Work out the finished part from the listing and answer in its coordinate system (mm). Face numbers are marked on the shaded views. Coordinates: 2 decimals unless noted, no trailing zeros. Order: outer loops, then holes, each group sorted by start corner. A loop starts at its lowest first (then second) coordinate and runs counter-clockwise, first axis right, second up. Notation, with made-up numbers: (71.25, -39.5) - (114.25, -39.5) arc R31 ccw to (114.25, -10.5) - close; hole circle Ø1 at (3.5, 16). An arc over 180 degrees is marked (long way). Answer as a JSON object with one key per item and string values. Group by question number.
1) Find the intervals of material crossed by line 1 along Y through (x, z) = (94.15, 13.65); line 2 along X through (y, z) = (-47, 10.75); line 3 along Y through (x, z) = (-94.15, 6.5), in increasing order.
2) Each of these flat-tipped pins is pushed along its axis until it touches: P1, Ø2, axis at x = -94.5, y = 53, coming from the +Z side; P2, Ø12, axis at x = 78, y = -17.5, coming from the -Z side; P3, Ø6.5, axis at x = 94.15, y = -54, coming from the -Z side. Where does it stop, or does it pass through?
3) Section C-C (z = 8) is taken. Count the separate pieces of the cut face and the enclosed holes in it, plus the area to 3 significant figures.
4) Section B-B (y = -26) is taken. Give the vertices of the cut face in (x, z).
5) Section A-A (x = 37) is taken. Give the vertices of the cut face in (y, z), plus the area to 3 significant figures.
6) The mould has two halves that part along X. Classify the marked faces 1 and 2: released by +X, released by -X, zero draft, split by the parting line, or undercut.
from build123d import *

# Parameters (mm, degrees)
SKETCH1_R           = 2
BOSS_EXTRUDE1_DEPTH = 15.2
SKETCH2_R           = 3.75
CUT_EXTRUDE1_DEPTH  = 2.9
FILLET1_R           = 1
CUT_EXTRUDE2_DEPTH  = 11.2
BOSS_EXTRUDE2_DEPTH = 1
CUT_EXTRUDE3_DEPTH  = 2.5
CUT_EXTRUDE4_DEPTH  = 11.2


with BuildPart() as part:
    # Sketch1 → Boss-Extrude1 (new body)
    with BuildSketch(Plane.XY):
        with BuildLine():
            Line((-95, -60), (95, -60))
            ThreePointArc((95, -60), (98.535533906, -58.535533906), (100, -55))
            Line((100, -55), (100, 55))
            ThreePointArc((100, 55), (98.535533906, 58.535533906), (95, 60))
            Line((95, 60), (-95, 60))
            ThreePointArc((-95, 60), (-98.535533906, 58.535533906), (-100, 55))
            Line((-100, 55), (-100, -55))
            ThreePointArc((-100, -55), (-98.535533906, -58.535533906), (-95, -60))
        make_face()
        with Locations((94.15, -54)):
            Circle(SKETCH1_R, mode=Mode.SUBTRACT)
        with Locations((94.15, 54)):
            Circle(SKETCH1_R, mode=Mode.SUBTRACT)
        with Locations((-94.15, 54)):
            Circle(SKETCH1_R, mode=Mode.SUBTRACT)
        with Locations((-94.15, -54)):
            Circle(SKETCH1_R, mode=Mode.SUBTRACT)
    extrude(amount=BOSS_EXTRUDE1_DEPTH)

    # Sketch2 → Cut-Extrude1 (cut)
    with BuildSketch(Plane.XY.offset(15.2)):
        with Locations((-94.15, 54)):
            Circle(SKETCH2_R)
        with Locations((94.15, 54)):
            Circle(SKETCH2_R)
        with Locations((94.15, -54)):
            Circle(SKETCH2_R)
        with Locations((-94.15, -54)):
            Circle(SKETCH2_R)
    extrude(amount=-CUT_EXTRUDE1_DEPTH, mode=Mode.SUBTRACT)

    # Fillet1
    fillet1_edges = [part.edges().sort_by_distance(p)[0] for p in [
        (98.535533906, -58.535533906, 15.2),
        (100, 0, 15.2),
        (98.535533906, 58.535533906, 15.2),
        (0, 60, 15.2),
        (-98.535533906, 58.535533906, 15.2),
        (-100, 0, 15.2),
        (-98.535533906, -58.535533906, 15.2),
        (0, -60, 15.2),
    ]]
    fillet(fillet1_edges, radius=FILLET1_R)

    # Sketch3 → Cut-Extrude2 (cut)
    with BuildSketch(Plane(origin=(0, 0, 0), x_dir=(-1, 0, 0), z_dir=(0, 0, -1))):
        with BuildLine():
            Line((86.35, -52.7), (86.35, -42.7))
            ThreePointArc((86.35, -42.7), (87.960912703, -38.810912703), (91.85, -37.2))
            Line((91.85, -37.2), (92.7, -37.2))
            ThreePointArc((92.7, -37.2), (94.467766953, -36.467766953), (95.2, -34.7))
            Line((95.2, -34.7), (95.2, 34.7))
            ThreePointArc((95.2, 34.7), (94.467766953, 36.467766953), (92.7, 37.2))
            Line((92.7, 37.2), (91.85, 37.2))
            ThreePointArc((91.85, 37.2), (87.960912703, 38.810912703), (86.35, 42.7))
            Line((86.35, 42.7), (86.35, 52.7))
            ThreePointArc((86.35, 52.7), (85.617766953, 54.467766953), (83.85, 55.2))
            Line((83.85, 55.2), (-83.85, 55.2))
            ThreePointArc((-83.85, 55.2), (-85.617766953, 54.467766953), (-86.35, 52.7))
            Line((-86.35, 52.7), (-86.35, 42.7))
            ThreePointArc((-86.35, 42.7), (-87.960912703, 38.810912703), (-91.85, 37.2))
            Line((-91.85, 37.2), (-92.7, 37.2))
            ThreePointArc((-92.7, 37.2), (-94.467766953, 36.467766953), (-95.2, 34.7))
            Line((-95.2, 34.7), (-95.2, -34.7))
            ThreePointArc((-95.2, -34.7), (-94.467766953, -36.467766953), (-92.7, -37.2))
            Line((-92.7, -37.2), (-91.85, -37.2))
            ThreePointArc((-91.85, -37.2), (-87.960912703, -38.810912703), (-86.35, -42.7))
            Line((-86.35, -42.7), (-86.35, -52.7))
            ThreePointArc((-86.35, -52.7), (-85.617766953, -54.467766953), (-83.85, -55.2))
            Line((-83.85, -55.2), (83.85, -55.2))
            ThreePointArc((83.85, -55.2), (85.617766953, -54.467766953), (86.35, -52.7))
        make_face()
    extrude(amount=-CUT_EXTRUDE2_DEPTH, mode=Mode.SUBTRACT)

    # Sketch4 → Boss-Extrude2 (add)
    with BuildSketch(Plane(origin=(0, 0, 0), x_dir=(-1, 0, 0), z_dir=(0, 0, -1))):
        with BuildLine():
            Line((-83.85, -56.2), (83.85, -56.2))
            ThreePointArc((83.85, -56.2), (86.324873734, -55.174873734), (87.35, -52.7))
            Line((87.35, -52.7), (87.35, -42.7))
            ThreePointArc((87.35, -42.7), (88.668019485, -39.518019485), (91.85, -38.2))
            Line((91.85, -38.2), (92.7, -38.2))
            ThreePointArc((92.7, -38.2), (95.174873734, -37.174873734), (96.2, -34.7))
            Line((96.2, -34.7), (96.2, 34.7))
            ThreePointArc((96.2, 34.7), (95.174873734, 37.174873734), (92.7, 38.2))
            Line((92.7, 38.2), (91.85, 38.2))
            ThreePointArc((91.85, 38.2), (88.668019485, 39.518019485), (87.35, 42.7))
            Line((87.35, 42.7), (87.35, 52.7))
            ThreePointArc((87.35, 52.7), (86.324873734, 55.174873734), (83.85, 56.2))
            Line((83.85, 56.2), (-83.85, 56.2))
            ThreePointArc((-83.85, 56.2), (-86.324873734, 55.174873734), (-87.35, 52.7))
            Line((-87.35, 52.7), (-87.35, 42.7))
            ThreePointArc((-87.35, 42.7), (-88.668019485, 39.518019485), (-91.85, 38.2))
            Line((-91.85, 38.2), (-92.7, 38.2))
            ThreePointArc((-92.7, 38.2), (-95.174873734, 37.174873734), (-96.2, 34.7))
            Line((-96.2, 34.7), (-96.2, -34.7))
            ThreePointArc((-96.2, -34.7), (-95.174873734, -37.174873734), (-92.7, -38.2))
            Line((-92.7, -38.2), (-91.85, -38.2))
            ThreePointArc((-91.85, -38.2), (-88.668019485, -39.518019485), (-87.35, -42.7))
            Line((-87.35, -42.7), (-87.35, -52.7))
            ThreePointArc((-87.35, -52.7), (-86.324873734, -55.174873734), (-83.85, -56.2))
        make_face()
        with BuildLine():
            Line((86.35, -52.7), (86.35, -42.7))
            ThreePointArc((86.35, -42.7), (87.960912703, -38.810912703), (91.85, -37.2))
            Line((91.85, -37.2), (92.7, -37.2))
            ThreePointArc((92.7, -37.2), (94.467766953, -36.467766953), (95.2, -34.7))
            Line((95.2, -34.7), (95.2, 34.7))
            ThreePointArc((95.2, 34.7), (94.467766953, 36.467766953), (92.7, 37.2))
            Line((92.7, 37.2), (91.85, 37.2))
            ThreePointArc((91.85, 37.2), (87.960912703, 38.810912703), (86.35, 42.7))
            Line((86.35, 42.7), (86.35, 52.7))
            ThreePointArc((86.35, 52.7), (85.617766953, 54.467766953), (83.85, 55.2))
            Line((83.85, 55.2), (-83.85, 55.2))
            ThreePointArc((-83.85, 55.2), (-85.617766953, 54.467766953), (-86.35, 52.7))
            Line((-86.35, 52.7), (-86.35, 42.7))
            ThreePointArc((-86.35, 42.7), (-87.960912703, 38.810912703), (-91.85, 37.2))
            Line((-91.85, 37.2), (-92.7, 37.2))
            ThreePointArc((-92.7, 37.2), (-94.467766953, 36.467766953), (-95.2, 34.7))
            Line((-95.2, 34.7), (-95.2, -34.7))
            ThreePointArc((-95.2, -34.7), (-94.467766953, -36.467766953), (-92.7, -37.2))
            Line((-92.7, -37.2), (-91.85, -37.2))
            ThreePointArc((-91.85, -37.2), (-87.960912703, -38.810912703), (-86.35, -42.7))
            Line((-86.35, -42.7), (-86.35, -52.7))
            ThreePointArc((-86.35, -52.7), (-85.617766953, -54.467766953), (-83.85, -55.2))
            Line((-83.85, -55.2), (83.85, -55.2))
            ThreePointArc((83.85, -55.2), (85.617766953, -54.467766953), (86.35, -52.7))
        make_face(mode=Mode.SUBTRACT)
    extrude(amount=BOSS_EXTRUDE2_DEPTH)

    # Sketch5 → Cut-Extrude3 (cut)
    with BuildSketch(Plane(origin=(0, 0, 0), x_dir=(-1, 0, 0), z_dir=(0, 0, -1))):
        with BuildLine():
            Line((92.7, 40.2), (91.85, 40.2))
            ThreePointArc((91.85, 40.2), (90.082233047, 40.932233047), (89.35, 42.7))
            Line((89.35, 42.7), (89.35, 52.7))
            ThreePointArc((89.35, 52.7), (87.739087297, 56.589087297), (83.85, 58.2))
            Line((83.85, 58.2), (-83.85, 58.2))
            ThreePointArc((-83.85, 58.2), (-87.739087297, 56.589087297), (-89.35, 52.7))
            Line((-89.35, 52.7), (-89.35, 42.7))
            ThreePointArc((-89.35, 42.7), (-90.082233047, 40.932233047), (-91.85, 40.2))
            Line((-91.85, 40.2), (-92.7, 40.2))
            ThreePointArc((-92.7, 40.2), (-96.589087297, 38.589087297), (-98.2, 34.7))
            Line((-98.2, 34.7), (-98.2, -34.7))
            ThreePointArc((-98.2, -34.7), (-96.589087297, -38.589087297), (-92.7, -40.2))
            Line((-92.7, -40.2), (-91.85, -40.2))
            ThreePointArc((-91.85, -40.2), (-90.082233047, -40.932233047), (-89.35, -42.7))
            Line((-89.35, -42.7), (-89.35, -52.7))
            ThreePointArc((-89.35, -52.7), (-87.739087297, -56.589087297), (-83.85, -58.2))
            Line((-83.85, -58.2), (83.85, -58.2))
            ThreePointArc((83.85, -58.2), (87.739087297, -56.589087297), (89.35, -52.7))
            Line((89.35, -52.7), (89.35, -42.7))
            ThreePointArc((89.35, -42.7), (90.082233047, -40.932233047), (91.85, -40.2))
            Line((91.85, -40.2), (92.7, -40.2))
            ThreePointArc((92.7, -40.2), (96.589087297, -38.589087297), (98.2, -34.7))
            Line((98.2, -34.7), (98.2, 34.7))
            ThreePointArc((98.2, 34.7), (96.589087297, 38.589087297), (92.7, 40.2))
        make_face()
        with BuildLine():
            Line((87.35, 42.7), (87.35, 52.7))
            ThreePointArc((87.35, 52.7), (86.324873734, 55.174873734), (83.85, 56.2))
            Line((83.85, 56.2), (-83.85, 56.2))
            ThreePointArc((-83.85, 56.2), (-86.324873734, 55.174873734), (-87.35, 52.7))
            Line((-87.35, 52.7), (-87.35, 42.7))
            ThreePointArc((-87.35, 42.7), (-88.668019485, 39.518019485), (-91.85, 38.2))
            Line((-91.85, 38.2), (-92.7, 38.2))
            ThreePointArc((-92.7, 38.2), (-95.174873734, 37.174873734), (-96.2, 34.7))
            Line((-96.2, 34.7), (-96.2, -34.7))
            ThreePointArc((-96.2, -34.7), (-95.174873734, -37.174873734), (-92.7, -38.2))
            Line((-92.7, -38.2), (-91.85, -38.2))
            ThreePointArc((-91.85, -38.2), (-88.668019485, -39.518019485), (-87.35, -42.7))
            Line((-87.35, -42.7), (-87.35, -52.7))
            ThreePointArc((-87.35, -52.7), (-86.324873734, -55.174873734), (-83.85, -56.2))
            Line((-83.85, -56.2), (83.85, -56.2))
            ThreePointArc((83.85, -56.2), (86.324873734, -55.174873734), (87.35, -52.7))
            Line((87.35, -52.7), (87.35, -42.7))
            ThreePointArc((87.35, -42.7), (88.668019485, -39.518019485), (91.85, -38.2))
            Line((91.85, -38.2), (92.7, -38.2))
            ThreePointArc((92.7, -38.2), (95.174873734, -37.174873734), (96.2, -34.7))
            Line((96.2, -34.7), (96.2, 34.7))
            ThreePointArc((96.2, 34.7), (95.174873734, 37.174873734), (92.7, 38.2))
            Line((92.7, 38.2), (91.85, 38.2))
            ThreePointArc((91.85, 38.2), (88.668019485, 39.518019485), (87.35, 42.7))
        make_face(mode=Mode.SUBTRACT)
    extrude(amount=-CUT_EXTRUDE3_DEPTH, mode=Mode.SUBTRACT)

    # Sketch6 → Cut-Extrude4 (cut)
    with BuildSketch(Plane(origin=(0, 0, 0), x_dir=(-1, 0, 0), z_dir=(0, 0, -1))):
        with BuildLine():
            Line((-97.6, 49.275595276), (-97.6, 39.838093031))
            ThreePointArc((-97.6, 39.838093031), (-95.339085019, 41.291299588), (-92.7, 41.8))
            Line((-92.7, 41.8), (-91.85, 41.8))
            ThreePointArc((-91.85, 41.8), (-91.213603897, 42.063603897), (-90.95, 42.7))
            Line((-90.95, 42.7), (-90.95, 49.102806926))
            ThreePointArc((-90.95, 49.102806926), (-94.301950497, 48.151973748), (-97.6, 49.275595276))
        make_face()
        with BuildLine():
            Line((-97.6, -39.838093031), (-97.6, -49.275595276))
            ThreePointArc((-97.6, -49.275595276), (-94.301950497, -48.151973748), (-90.95, -49.102806926))
            Line((-90.95, -49.102806926), (-90.95, -42.7))
            ThreePointArc((-90.95, -42.7), (-91.213603897, -42.063603897), (-91.85, -41.8))
            Line((-91.85, -41.8), (-92.7, -41.8))
            ThreePointArc((-92.7, -41.8), (-95.339085019, -41.291299588), (-97.6, -39.838093031))
        make_face()
        with BuildLine():
            Line((90.95, -42.7), (90.95, -49.102806926))
            ThreePointArc((90.95, -49.102806926), (94.301950497, -48.151973748), (97.6, -49.275595276))
            Line((97.6, -49.275595276), (97.6, -39.838093031))
            ThreePointArc((97.6, -39.838093031), (95.339085019, -41.291299588), (92.7, -41.8))
            Line((92.7, -41.8), (91.85, -41.8))
            ThreePointArc((91.85, -41.8), (91.213603897, -42.063603897), (90.95, -42.7))
        make_face()
        with BuildLine():
            ThreePointArc((92.7, 41.8), (95.339085019, 41.291299588), (97.6, 39.838093031))
            Line((97.6, 39.838093031), (97.6, 49.275595276))
            ThreePointArc((97.6, 49.275595276), (94.301950497, 48.151973748), (90.95, 49.102806926))
            Line((90.95, 49.102806926), (90.95, 42.7))
            ThreePointArc((90.95, 42.7), (91.213603897, 42.063603897), (91.85, 41.8))
            Line((91.85, 41.8), (92.7, 41.8))
        make_face()
    extrude(amount=-CUT_EXTRUDE4_DEPTH, mode=Mode.SUBTRACT)


solid = part.part
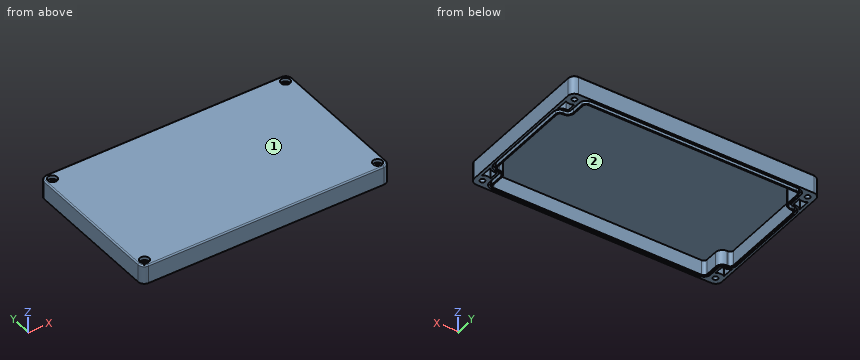
Report:
{
 "1": {"line 1": "y = -60 to -57.75, -50.25 to 50.25, 57.75 to 60", "line 2": "x = -100 to -97.6, -90.95 to -86.35, 86.35 to 90.95, 97.6 to 100", "line 3": "y = -60 to -56, -52 to -48.15, -41.65 to -36.74, 36.74 to 41.65, 48.15 to 52, 56 to 60"},
 "2": {"P1": "stops at z = 12.3", "P2": "stops at z = 11.2", "P3": "stops at z = 0"},
 "3": {"separate pieces": "1", "enclosed holes": "9", "area": "3,340 mm²"},
 "4": {"outline": "(-100, 0) - (-98.2, 0) - (-98.2, 2.5) - (-96.2, 2.5) - (-96.2, -1) - (-95.2, -1) - (-95.2, 11.2) - (95.2, 11.2) - (95.2, -1) - (96.2, -1) - (96.2, 2.5) - (98.2, 2.5) - (98.2, 0) - (100, 0) - (100, 14.2) arc R1 ccw to (99, 15.2) - (-99, 15.2) arc R1 ccw to (-100, 14.2) - close"},
 "5": {"outline": "(-60, 0) - (-58.2, 0) - (-58.2, 2.5) - (-56.2, 2.5) - (-56.2, -1) - (-55.2, -1) - (-55.2, 11.2) - (55.2, 11.2) - (55.2, -1) - (56.2, -1) - (56.2, 2.5) - (58.2, 2.5) - (58.2, 0) - (60, 0) - (60, 14.2) arc R1 ccw to (59, 15.2) - (-59, 15.2) arc R1 ccw to (-60, 14.2) - close", "area": "579 mm²"},
 "6": {"face 1": "zero draft", "face 2": "undercut"}
}
